Input: part model. Units: mm. Frame: model coordinates. A direction names the side the tool comes from. Coordinates: 2 decimals unless noted, no trailing zeros. One line per item, written item: value. Start each with the question number.
from build123d import *
from OCP.BRepFilletAPI import BRepFilletAPI_MakeChamfer

# Parameters (mm, degrees)
SKETCH1_R                      = 25
BOSS_EXTRUDE1_DEPTH            = 5
SKETCH2_W                      = 10
SKETCH2_H                      = 20
BOSS_EXTRUDE2_DEPTH            = 10
FILLET1_R                      = 10
FILLET2_R                      = 5
SKETCH3_R                      = 1.75
CUT_EXTRUDE1_DEPTH             = 20
SKETCH4_W                      = 5.7
SKETCH4_H                      = 3
CUT_EXTRUDE2_DEPTH             = 8
CIRPATTERN1_COUNT              = 3
SKETCH5_R                      = 1.75
CUT_EXTRUDE3_DEPTH             = 50.005657282
SKETCH7_R                      = 7.5
CUT_EXTRUDE5_DEPTH             = 50.005657282
SKETCH8_R                      = 3.5
BOSS_EXTRUDE3_DEPTH            = 2
CHAMFER1_SIZE2                 = 1.154700538
CHAMFER1_SIZE                  = 2
SKETCH9_R                      = 1.75
CUT_EXTRUDE6_DEPTH             = 2
CIRPATTERN2_COUNT              = 3
CHAMFER1_OF_CIRPATTERN2_SIZE   = 2
CHAMFER1_OF_CIRPATTERN2_SIZE_2 = 1.154700538
SKETCH10_R                     = 1.75
CUT_EXTRUDE7_DEPTH             = 2
SKETCH11_R                     = 1.75
CUT_EXTRUDE8_DEPTH             = 2
CUT_EXTRUDE9_DEPTH             = 3


with BuildPart() as part:
    # Sketch1 → Boss-Extrude1 (new, symmetric)
    with BuildSketch(Plane(origin=(0, 0, 0), x_dir=(1, 0, 0), z_dir=(0, 1, 0))):
        with Locations(Location((0, 0, 0), (0, 0, 270))):
            Circle(SKETCH1_R)
    extrude(amount=BOSS_EXTRUDE1_DEPTH, both=True)

    # Sketch2 → Boss-Extrude2 (add)
    with BuildSketch(Plane(origin=(0, 5, 0), x_dir=(1, 0, 0), z_dir=(0, 1, 0))):
        Polygon((15.490381057, -3.169872981), (10.490381057, -11.830127019), (27.810889132, -21.830127019), (32.810889132, -13.169872981), align=None)
        with Locations((0, 25)):
            Rectangle(SKETCH2_W, SKETCH2_H)
        Polygon((-10.490381057, -11.830127019), (-15.490381057, -3.169872981), (-32.810889132, -13.169872981), (-27.810889132, -21.830127019), align=None)
    extrude(amount=-BOSS_EXTRUDE2_DEPTH)

    # Fillet1
    fillet1_edges = [part.edges().sort_by_distance(p)[0] for p in [
        (5, 0, -24.494897428),
        (-5, 0, -24.494897428),
        (18.713203436, 0, 16.577575733),
        (23.713203436, 0, 7.917321695),
        (-23.713203436, 0, 7.917321695),
        (-18.713203436, 0, 16.577575733),
    ]]
    fillet(fillet1_edges, radius=FILLET1_R)

    # Fillet2
    fillet2_edges = [part.edges().sort_by_distance(p)[0] for p in [
        (-5, 5, -33.311388301),
        (-6.548457453, 5, -26.277551763),
        (-6.548457453, -5, -26.277551763),
        (-31.348508504, 5, 12.325567131),
        (-26.031256103, -5, 7.467645372),
        (-26.031256103, 5, 7.467645372),
        (31.348508504, 5, 12.325567131),
        (26.031256103, 5, 7.467645372),
        (26.031256103, -5, 7.467645372),
        (5, 5, -33.311388301),
        (6.548457453, -5, -26.277551763),
        (6.548457453, 5, -26.277551763),
        (-26.348508504, 5, 20.985821169),
        (-19.48279865, 5, 18.809906391),
        (-19.48279865, -5, 18.809906391),
        (26.348508504, 5, 20.985821169),
        (19.48279865, -5, 18.809906391),
        (19.48279865, 5, 18.809906391),
        (-21.650635095, 5, -12.5),
        (-21.650635095, -5, -12.5),
        (21.650635095, 5, -12.5),
        (21.650635095, -5, -12.5),
        (0, 5, 25),
        (0, -5, 25),
        (31.348508504, -5, 12.325567131),
        (5, -5, -33.311388301),
        (-26.348508504, -5, 20.985821169),
        (26.348508504, -5, 20.985821169),
        (-31.348508504, -5, 12.325567131),
        (-5, -5, -33.311388301),
    ]]
    fillet(fillet2_edges, radius=FILLET2_R - 0.0001)  # a hair under: the kernel refuses the full size

    # Sketch3 → Cut-Extrude1 (cut)
    with BuildSketch(Plane(origin=(0, 0, -35), x_dir=(-1, 0, 0), z_dir=(0, 0, -1))):
        Circle(SKETCH3_R)
    cut_extrude1 = extrude(amount=-CUT_EXTRUDE1_DEPTH, mode=Mode.SUBTRACT)

    # Sketch4 → Cut-Extrude2 (cut)
    with BuildSketch(Plane.XZ.offset(5)):
        with Locations((0, -20)):
            Rectangle(SKETCH4_W, SKETCH4_H)
    cut_extrude2 = extrude(amount=-CUT_EXTRUDE2_DEPTH, mode=Mode.SUBTRACT)

    # CirPattern1: Cut-Extrude1, Cut-Extrude2 ×3 about axis
    cirpattern1_axis = Axis((0, 0, 0), (0, 1, 0))
    add([cut_extrude1.rotate(cirpattern1_axis, i * 360 / CIRPATTERN1_COUNT) for i in range(1, CIRPATTERN1_COUNT)], mode=Mode.SUBTRACT)
    add([cut_extrude2.rotate(cirpattern1_axis, i * 360 / CIRPATTERN1_COUNT) for i in range(1, CIRPATTERN1_COUNT)], mode=Mode.SUBTRACT)

    # Sketch5 → Cut-Extrude3 (cut, through all)
    with BuildSketch(Plane(origin=(0, 5, 0), x_dir=(1, 0, 0), z_dir=(0, 1, 0))):
        with Locations(Location((-12.990381057, 7.5, 0), (0, 0, 270))):
            Circle(SKETCH5_R)
        with Locations(Location((12.990381057, 7.5, 0), (0, 0, 270))):
            Circle(SKETCH5_R)
        with Locations(Location((0, -15, 0), (0, 0, 270))):
            Circle(SKETCH5_R)
    extrude(amount=-CUT_EXTRUDE3_DEPTH, mode=Mode.SUBTRACT)

    # Sketch7 → Cut-Extrude5 (cut, through all)
    with BuildSketch(Plane(origin=(0, 5, 0), x_dir=(1, 0, 0), z_dir=(0, 1, 0))):
        with Locations(Location((0, 0, 0), (0, 0, 270))):
            Circle(SKETCH7_R)
    extrude(amount=-CUT_EXTRUDE5_DEPTH, mode=Mode.SUBTRACT)

    # Sketch8 → Boss-Extrude3 (add)
    with BuildSketch(Plane(origin=(30.310889132, 0, 17.5), x_dir=(0.4999999999999999, 0, -0.8660254037844386), z_dir=(0.8660254037844387, 0, 0.49999999999999994))):
        Circle(SKETCH8_R)
    boss_extrude3 = extrude(amount=BOSS_EXTRUDE3_DEPTH)

    # Chamfer1
    chamfer1_edges = [part.edges().sort_by_distance(p)[0] for p in [
        (30.29293994, 0, 21.531088913),
    ]]
    chamfer1_side = [part.faces().sort_by_distance(p)[0] for p in [
        (30.27293994, 0, 21.519541908),
    ]]
    chamfer(chamfer1_edges, length=CHAMFER1_SIZE - 0.0001, length2=CHAMFER1_SIZE2 - 0.0001, reference=chamfer1_side[0])  # a hair under: the kernel refuses the full size

    # Sketch9 → Cut-Extrude6 (cut)
    with BuildSketch(Plane(origin=(32.04293994, 0, 18.5), x_dir=(0.49999999999999983, 0, -0.8660254037844387), z_dir=(0.8660254037844387, 0, 0.49999999999999983))):
        Circle(SKETCH9_R)
    extrude(amount=-CUT_EXTRUDE6_DEPTH, mode=Mode.SUBTRACT)

    # CirPattern2: Boss-Extrude3 ×3 about axis
    cirpattern2_axis = Axis((0, 0, 0), (0, 1, 0))
    for i in range(1, CIRPATTERN2_COUNT):
        add(boss_extrude3.rotate(cirpattern2_axis, i * 360 / CIRPATTERN2_COUNT))

    # Chamfer1 of CirPattern2
    chamfer1_of_cirpattern2_edges_1 = [part.edges().sort_by_distance(p)[0] for p in [
        (3.5, 0, -37),
    ]]
    chamfer1_of_cirpattern2_side_1 = [part.faces().sort_by_distance(p)[0] for p in [
        (3.5, 0, -36.976905989),
    ]]
    chamfer1_of_cirpattern2_edges_2 = [part.edges().sort_by_distance(p)[0] for p in [
        (-33.79293994, 0, 15.468911087),
    ]]
    chamfer1_of_cirpattern2_side_2 = [part.faces().sort_by_distance(p)[0] for p in [
        (-33.77293994, 0, 15.457364081),
    ]]
    chamfer1_of_cirpattern2 = BRepFilletAPI_MakeChamfer(part.part.solid().wrapped)
    for e in chamfer1_of_cirpattern2_edges_1:
        chamfer1_of_cirpattern2.Add(CHAMFER1_OF_CIRPATTERN2_SIZE - 0.0001, CHAMFER1_OF_CIRPATTERN2_SIZE_2 - 0.0001, e.wrapped, chamfer1_of_cirpattern2_side_1[0].wrapped)
    for e in chamfer1_of_cirpattern2_edges_2:
        chamfer1_of_cirpattern2.Add(CHAMFER1_OF_CIRPATTERN2_SIZE - 0.0001, CHAMFER1_OF_CIRPATTERN2_SIZE_2 - 0.0001, e.wrapped, chamfer1_of_cirpattern2_side_2[0].wrapped)
    add(Compound.cast(chamfer1_of_cirpattern2.Shape()), mode=Mode.REPLACE)  # a hair under: the kernel refuses the full size

    # Sketch10 → Cut-Extrude7 (cut)
    with BuildSketch(Plane(origin=(-32.04293994, 0, 18.5), x_dir=(0.4999999999999961, 0, 0.8660254037844409), z_dir=(-0.8660254037844409, 0, 0.4999999999999961))):
        Circle(SKETCH10_R)
    extrude(amount=-CUT_EXTRUDE7_DEPTH, mode=Mode.SUBTRACT)

    # Sketch11 → Cut-Extrude8 (cut)
    with BuildSketch(Plane(origin=(0, 0, -37), x_dir=(-1, 0, 0), z_dir=(0, 0, -1))):
        Circle(SKETCH11_R)
    extrude(amount=-CUT_EXTRUDE8_DEPTH, mode=Mode.SUBTRACT)

    # Sketch12 → Cut-Extrude9 (cut)
    with BuildSketch(Plane.XZ.offset(5)):
        Polygon((12.990381057, -10.790896534), (15.840381057, -9.145448267), (15.840381057, -5.854551733), (12.990381057, -4.209103466), (10.140381057, -5.854551733), (10.140381057, -9.145448267), align=None)
        Polygon((-15.840381057, -5.854551733), (-15.840381057, -9.145448267), (-12.990381057, -10.790896534), (-10.140381057, -9.145448267), (-10.140381057, -5.854551733), (-12.990381057, -4.209103466), align=None)
        Polygon((2.85, 16.645448267), (0, 18.290896534), (-2.85, 16.645448267), (-2.85, 13.354551733), (0, 11.709103466), (2.85, 13.354551733), align=None)
    extrude(amount=-CUT_EXTRUDE9_DEPTH, mode=Mode.SUBTRACT)


solid = part.part
1) Pin query (flat end, axial travel): pin 1 Ø1.7 at (x, z) = (-13, -8) entering from -Y; pin 2 Ø1.7 at (x, y) = (1, -0.5) entering from +Z; pin 3 Ø2.5 at (y, z) = (-4, 15.5) entering from -X; pin 4 Ø1.5 at (y, z) = (0.5, -9) entering from -X. Return the tip coordinate at first contact, or that it passes through.
2) Access query for faces 4 (the flat face through (-15.84, -4, -7)), 5 (the cylindrical face through (3, 4, -33)), 6 (the cylindrical face through (-1.617, -0.67, -29.358)), 7 (the cylindrical face through (14.466, 1.549, -6.559)). Directions: +Z, -Z, +X, -X, +Y, -Y. A direction counts if a zero-diameter tool reaches every point of the face in a straight line with its end or side. Return the directions, or none.
3) Ray query, line 1 along X through (y, z) = (2.5, 12); line 2 along Z through (x, y) = (-1, 2); line 3 along X through (y, z) = (-1, 0). Return the intervals inside material, ascending. Write a range as from..to.
4) Mould query, pull axis Z, two halves, no side actions, for faces 1 (the cylindrical face through (30.576, 3.574, 13.616)), 2 (the cylindrical face through (-1.617, -0.67, -16.774)), 3 (the cylindrical face through (-26.299, 0.077, 13.165)). Classes: +Z half, -Z half, draft (parallel to the pull), parting line (faces both ways), or undercut.
Entries:
1. pin 1: passes through
1. pin 2: stops at z = 25
1. pin 3: stops at x = -32.12
1. pin 4: stops at x = -23.58
2. face 4: -Y
2. face 5: -Z, +X, +Y
2. face 6: -Z
2. face 7: +Y, -Y
3. line 1: x = -29.45..-17.9, -15.08..15.08, 17.9..29.45
3. line 2: z = -37..-21.5, -18.5..-7.43, 7.43..13.56, 16.44..24.56
3. line 3: x = -24.9..-7.5, 7.5..24.9
4. face 1: -Z half
4. face 2: draft
4. face 3: undercut
